Design review of the part built by this model. Coordinates are the model's own, in mm. Give positions to 0.01 mm unless a question says otherwise; leave off trailing zeros. Write each question's results on one line, items separated by ' | '.
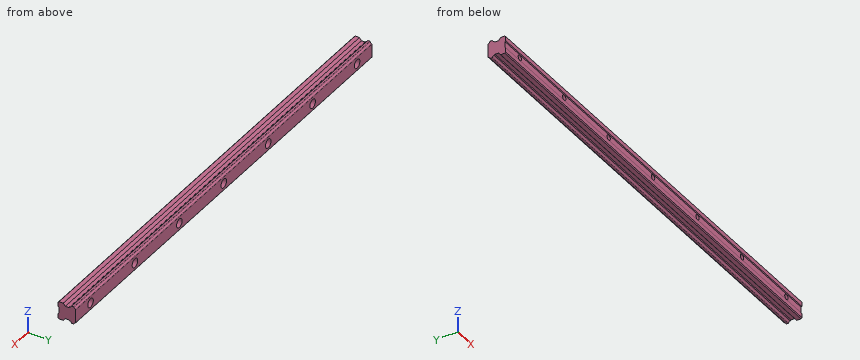
from build123d import *

# Parameters (mm, degrees)
SKETCH_1_W             = 15
SKETCH_1_H             = 15
EXTRUDE_1_DEPTH        = 200
CHAMFER_1_SIZE         = 0.75
SKETCH_3_R             = 3.74995
CUT_EXTRUDE_2_DEPTH    = 5.3
SKETCH_4_R             = 2.25
CUT_EXTRUDE_3_DEPTH    = 201.375497504
PATTERN_LINEAR_1_COUNT = 7
PATTERN_LINEAR_1_PITCH = 60
CUT_EXTRUDE_4_DEPTH    = 401.140600289
CUT_EXTRUDE_5_DEPTH    = 401.140600289
FILLET_1_R             = 0.5
CUT_EXTRUDE_6_DEPTH    = 401.140600289


with BuildPart() as part:
    # 草图1 → 凸台-拉伸1 (new, symmetric)
    with BuildSketch(Plane(origin=(0, 0, 0), x_dir=(0, 0, -1), z_dir=(1, 0, 0))):
        Rectangle(SKETCH_1_W, SKETCH_1_H)
    extrude(amount=EXTRUDE_1_DEPTH, both=True)

    # 倒角1
    chamfer_1_edges = [part.edges().sort_by_distance(p)[0] for p in [
        (0, -7.5, -7.5),
        (0, -7.5, 7.5),
    ]]
    chamfer(chamfer_1_edges, length=CHAMFER_1_SIZE)

    # 草图3 → 切除-拉伸2 (cut)
    with BuildSketch(Plane(origin=(0, 7.5, 0), x_dir=(1, 0, 0), z_dir=(0, 1, 0))):
        with Locations(Location((-180, 0, 0), (0, 0, 270))):
            Circle(SKETCH_3_R)
    cut_extrude_2 = extrude(amount=-CUT_EXTRUDE_2_DEPTH, mode=Mode.SUBTRACT)

    # 草图4 → 切除-拉伸3 (cut, through all)
    with BuildSketch(Plane(origin=(0, 2.2, 0), x_dir=(1, 0, 0), z_dir=(0, 1, 0))):
        with Locations(Location((-180, 0, 0), (0, 0, 270))):
            Circle(SKETCH_4_R)
    cut_extrude_3 = extrude(amount=-CUT_EXTRUDE_3_DEPTH, mode=Mode.SUBTRACT)

    # 阵列(线性)1: 切除-拉伸2, 切除-拉伸3 ×7
    with Locations(*[(i * PATTERN_LINEAR_1_PITCH, 0, 0) for i in range(1, PATTERN_LINEAR_1_COUNT)]):
        add(cut_extrude_2, mode=Mode.SUBTRACT)
        add(cut_extrude_3, mode=Mode.SUBTRACT)

    # 草图2 → 切除-拉伸4 (cut, through all)
    with BuildSketch(Plane(origin=(200, 0, 0), x_dir=(0, 0, -1), z_dir=(1, 0, 0))):
        with BuildLine():
            Line((-7.5, 7.5), (-6, 7.5))
            ThreePointArc((-6, 7.5), (-6.439339828, 6.439339828), (-7.5, 6))
            Line((-7.5, 6), (-7.5, 7.5))
        make_face()
        with BuildLine():
            Line((7.5, 7.5), (7.5, 6))
            ThreePointArc((7.5, 6), (6.439339828, 6.439339828), (6, 7.5))
            Line((6, 7.5), (7.5, 7.5))
        make_face()
    extrude(amount=-CUT_EXTRUDE_4_DEPTH, mode=Mode.SUBTRACT)

    # 草图5 → 切除-拉伸5 (cut, through all)
    with BuildSketch(Plane(origin=(200, 0, 0), x_dir=(0, 0, -1), z_dir=(1, 0, 0))):
        with BuildLine():
            Line((-6, 2.25), (-5.4, 1.65))
            Line((-5.4, 1.65), (-5.4, -1.35))
            Line((-5.4, -1.35), (-7.5, -3.1))
            Line((-7.5, -3.1), (-7.5, 3.75))
            ThreePointArc((-7.5, 3.75), (-6.439339828, 3.310660172), (-6, 2.25))
        make_face()
        with BuildLine():
            Line((7.5, 3.75), (7.5, -3.1))
            Line((7.5, -3.1), (5.4, -1.35))
            Line((5.4, -1.35), (5.4, 1.65))
            Line((5.4, 1.65), (6, 2.25))
            ThreePointArc((6, 2.25), (6.439339828, 3.310660172), (7.5, 3.75))
        make_face()
    extrude(amount=-CUT_EXTRUDE_5_DEPTH, mode=Mode.SUBTRACT)

    # 圆角1
    fillet_1_edges = [part.edges().sort_by_distance(p)[0] for p in [
        (0, 3.75, -7.5),
        (0, 6, 7.5),
        (0, 7.5, 6),
        (0, 7.5, -6),
        (0, 6, -7.5),
        (0, 3.75, 7.5),
    ]]
    fillet(fillet_1_edges, radius=FILLET_1_R)

    # 草图6 → 切除-拉伸6 (cut, through all)
    with BuildSketch(Plane.ZY.offset(200)):
        Polygon((-3.1, -7.5), (-2.5, -6.9), (2.5, -6.9), (3.1, -7.5), align=None)
    extrude(amount=-CUT_EXTRUDE_6_DEPTH, mode=Mode.SUBTRACT)


solid = part.part
(1) Insertion check: P1, Ø8.5, axis at x = 60, z = 0, coming from the +Y side; P2, Ø0.9, axis at x = -58.5, y = -0.5, coming from the +Z side; P3, Ø2, axis at x = 120.5, z = 1, coming from the +Y side; P4, Ø3.5, axis at x = -1.5, z = 1, coming from the +Y side. Each pin has a flat end and moves straight along its axis. Give the tip position at first contact, or say it passes through.
Answers below:
P1: y = 7.5 | P2: z = 5.4 | P3: through | P4: y = 2.2
(2) Wall thickness on line 1 along Z through (x, y) = (0.5, -0.75); line 2 along Z through (x, y) = (-178, 2.25); line 3 along Y through (x, z) = (110.5, 1.75): over which ranges is each line inside the solid? List them lowest first. Write a range as from..to.
Answers below:
line 1: -5.4..-2.19, 2.19..5.4 | line 2: -6..-3.17, 3.17..6 | line 3: -6.9..7.5
(3) Take a section at B-B on z = 0. Count the separate pieces of the cut face and the enclosed holes in it, plus the area to 3 significant figures.
Answers below:
separate pieces: 8 | enclosed holes: 0 | area: 5,200 mm2
